```python
from build123d import *

# Parameters (mm, degrees)
SKETCH1_R           = 4.5
BOSS_EXTRUDE1_DEPTH = 4.5
SKETCH2_W           = 8
SKETCH2_H           = 10
BOSS_EXTRUDE2_DEPTH = 4.5
BOSS_EXTRUDE3_START = 4.5
SKETCH3_R           = 4.5
BOSS_EXTRUDE3_DEPTH = 4.5
FILLET3_R           = 5
FILLET4_R           = 5
SKETCH6_R           = 4.25
SKETCH6_R_2         = 1.5
BOSS_EXTRUDE4_DEPTH = 4.5
BOSS_EXTRUDE5_START = 4.5
SKETCH7_R           = 4.25
SKETCH7_R_2         = 1.5
BOSS_EXTRUDE5_DEPTH = 4.5
BOSS_EXTRUDE6_START = -2
SKETCH8_R           = 4.25
BOSS_EXTRUDE6_DEPTH = 2
BOSS_EXTRUDE7_START = -9.5
SKETCH9_R           = 4.5
BOSS_EXTRUDE7_DEPTH = 9.5


with BuildPart() as part:
    # Sketch1 → Boss-Extrude1 (new body)
    with BuildSketch(Plane.XY):
        with BuildLine():
            Line((-15, 17.5), (-15, -14.5))
            Line((-15, -14.5), (-12, -14.5))
            Line((-12, -14.5), (-12, -17.5))
            Line((-12, -17.5), (12, -17.5))
            Line((12, -17.5), (12, -14.5))
            Line((12, -14.5), (15, -14.5))
            Line((15, -14.5), (15, 17.5))
            ThreePointArc((15, 17.5), (0, 26.843803595), (-15, 17.5))
        make_face()
        with Locations((0, 17.5)):
            Circle(SKETCH1_R, mode=Mode.SUBTRACT)
    extrude(amount=-BOSS_EXTRUDE1_DEPTH)

    # Sketch2 → Boss-Extrude2 (add)
    with BuildSketch(Plane(origin=(0, -17.5, 0), x_dir=(1, 0, 0), z_dir=(0, 1, 0))):
        Polygon((-12, 4.5), (12, 4.5), (12, 0), (12, -3), (15, -3), (15, -12.000675804), (22.5, -12.000675804), (22.5, -15.000675804), (25.5, -15.000675804), (30, -15.000675804), (30, -39.000675804), (25.5, -39.000675804), (22.5, -39.000675804), (22.5, -42.000675804), (15, -42.000675804), (15, -47.001351609), (12, -47.001351609), (12, -50), (12, -54.5), (-12, -54.5), (-12, -50), (-12, -47), (-15, -47), (-15, -42.000675804), (-22.5, -42.000675804), (-22.5, -39.000675804), (-25.5, -39.000675804), (-30, -39.000675804), (-30, -15.000675804), (-25.5, -15.000675804), (-22.5, -15.000675804), (-22.5, -12.000675804), (-15, -12.000675804), (-15, -3), (-12, -3), (-12, 0), align=None)
        with Locations((0, -27.000675804)):
            Rectangle(SKETCH2_W, SKETCH2_H, mode=Mode.SUBTRACT)
    extrude(amount=-BOSS_EXTRUDE2_DEPTH)

    # Sketch3 → Boss-Extrude3 (add)
    with BuildSketch(Plane.XY.offset(50).offset(BOSS_EXTRUDE3_START)):
        with BuildLine():
            Line((-15, 17.5), (-15, -14.5))
            Line((-15, -14.5), (-12, -14.5))
            Line((-12, -14.5), (-12, -17.5))
            Line((-12, -17.5), (12, -17.5))
            Line((12, -17.5), (12, -14.5))
            Line((12, -14.5), (15, -14.5))
            Line((15, -14.5), (15, 17.5))
            ThreePointArc((15, 17.5), (0, 26.843803595), (-15, 17.5))
        make_face()
        with Locations((0, 17.5)):
            Circle(SKETCH3_R, mode=Mode.SUBTRACT)
    extrude(amount=-BOSS_EXTRUDE3_DEPTH)

    # Fillet3
    fillet3_edges = [part.edges().sort_by_distance(p)[0] for p in [
        (0, -22, 54.5),
    ]]
    fillet(fillet3_edges, radius=FILLET3_R)

    # Fillet4
    fillet4_edges = [part.edges().sort_by_distance(p)[0] for p in [
        (0, -22, -4.5),
    ]]
    fillet(fillet4_edges, radius=FILLET4_R)

    # Sketch6 → Boss-Extrude4 (add)
    with BuildSketch(Plane(origin=(-25.5, 0, 0), x_dir=(0, 0, -1), z_dir=(1, 0, 0))):
        Polygon((-15.000675804, -22), (-39.000675804, -22), (-39.000675804, -25), (-42.000675804, -25), (-42.000675804, -67), (-27.000675804, -75), (-12.000675804, -67), (-12.000675804, -25), (-15.000675804, -25), align=None)
        with Locations((-27.000675804, -49)):
            Circle(SKETCH6_R, mode=Mode.SUBTRACT)
        with Locations((-27.000675804, -61)):
            Circle(SKETCH6_R_2, mode=Mode.SUBTRACT)
    extrude(amount=-BOSS_EXTRUDE4_DEPTH)

    # Sketch7 → Boss-Extrude5 (add)
    with BuildSketch(Plane(origin=(25.5, 0, 0), x_dir=(0, 0, -1), z_dir=(1, 0, 0)).offset(BOSS_EXTRUDE5_START)):
        Polygon((-39.000675804, -22), (-39.000675804, -25), (-42.000675804, -25), (-42.000675804, -67), (-27.000675804, -75), (-12.000675804, -67), (-12.000675804, -25), (-15.000675804, -25), (-15.000675804, -22), align=None)
        with Locations((-27.000675804, -49)):
            Circle(SKETCH7_R, mode=Mode.SUBTRACT)
        with Locations((-27.000675804, -61)):
            Circle(SKETCH7_R_2, mode=Mode.SUBTRACT)
    extrude(amount=-BOSS_EXTRUDE5_DEPTH)

    # Sketch8 → Boss-Extrude6 (add)
    with BuildSketch(Plane.ZY.offset(30).offset(BOSS_EXTRUDE6_START)):
        with Locations(Location((27.000675804, -49, 0), (0, 0, 180))):
            Circle(SKETCH8_R)
    extrude(amount=BOSS_EXTRUDE6_DEPTH)

    # Sketch9 → Boss-Extrude7 (add)
    with BuildSketch(Plane(origin=(0, 0, 50), x_dir=(-1, 0, 0), z_dir=(0, 0, -1)).offset(BOSS_EXTRUDE7_START)):
        with Locations(Location((0, 17.5, 0), (0, 0, 180))):
            Circle(SKETCH9_R)
    extrude(amount=BOSS_EXTRUDE7_DEPTH)


solid = part.part
```
Read the model definition and answer for the solid it produces. Units are mm, in the model's axes. A direction names the side the tool comes from. Give positions to 0.01 mm unless a question says otherwise; leave off trailing zeros. Write each loop counter-clockwise with the first axis right and the second up, starting at its lowest first coordinate (ties: lowest second). Pieces come first, ordered by that corner, then holes. Notation, with made-up numbers: (32.25, 31) -> (63.25, 31) arc R13 ccw to (63.25, 43) -> close; hole circle Ø10 at (-11, -38.75). An arc over 180 degrees is marked (long way). Answer as a JSON object with one key per item and string values.
1) Section C-C on y = -23.5 is taken. Write down the section's boundary in (x, z).
Findings below:
{"outline": "(-30, 15) -> (-25.5, 15) -> (-25.5, 39) -> (-30, 39) -> close; (25.5, 15) -> (30, 15) -> (30, 39) -> (25.5, 39) -> close"}
2) Flat-ended cylindrical pins translate along their axes: pin 1 Ø4 at (y, z) = (-48.5, 28.5) entering from +X; pin 2 Ø3.5 at (x, y) = (-0.5, -19.5) entering from +Z; pin 3 Ø8 at (x, z) = (-10.5, 53) entering from +Y; pin 4 Ø4 at (x, y) = (23, -46.5) entering from +Z. Find the tip coordinate at first contact, or state that the pin passes through.
Findings below:
{"pin 1": "stops at x = -28", "pin 2": "stops at z = 54.44", "pin 3": "stops at y = 25.53", "pin 4": "passes through"}
3) Section D-D on z = 36 is taken. Write down the section's boundary in (x, y).
Findings below:
{"outline": "(-30, -70.2) -> (-25.5, -70.2) -> (-25.5, -22) -> (25.5, -22) -> (25.5, -70.2) -> (30, -70.2) -> (30, -17.5) -> (-30, -17.5) -> close"}
4) Section A-A on x = 0 is taken. Write down the section's boundary in (y, z), then the cut area to 3 significant figures.
Findings below:
{"outline": "(-22, 0.5) arc R5 ccw to (-17, -4.5) -> (13, -4.5) -> (13, 0) -> (-17.5, 0) -> (-17.5, 22) -> (-22, 22) -> close; (-22, 32) -> (-17.5, 32) -> (-17.5, 50) -> (26.84, 50) -> (26.84, 54.5) -> (22, 54.5) -> (22, 59.5) -> (13, 59.5) -> (13, 54.5) -> (-17, 54.5) arc R5 ccw to (-22, 49.5) -> close; (22, -4.5) -> (26.84, -4.5) -> (26.84, 0) -> (22, 0) -> close", "area": "613 mm^2"}
5) A tool of negligible diameter and unlimited length cuts with its end or side. For faces 4 (the flat face through (22.5, -20, 13)), 5 (the flat face through (-12, -18, -1)), 6 (the cylindrical face through (-26.73, -51.59, 30.37)), 7 (the flat face through (28, -25, 13)), 8 (the flat face through (-12, -18, 51)), from which of +Z, -Z, +X, -X, +Y, -Y can it reach the whole face along a straight path? Write none if from no direction.
Findings below:
{"face 4": "-Z, +X, +Y, -Y", "face 5": "-Z, -X, -Y", "face 6": "+X", "face 7": "-Z, +X, -X, +Y", "face 8": "+Z, -X, -Y"}
6) Straight lines are drawn through the part: probe 1 along X at (y, z) = (-48, 40); probe 2 along Z at (x, y) = (-4, -13); probe 3 along Z at (x, y) = (-27.35, -49). For each, find the intervals that lie inside material, in ascending order. Write a range as from..to.
Findings below:
{"probe 1": "x = -30..-25.5, 25.5..30", "probe 2": "z = -4.5..0, 50..54.5", "probe 3": "z = 12..22.75, 31.25..42"}
7) Section B-B on y = -57 is taken. Write down the section's boundary in (x, z).
Findings below:
{"outline": "(-30, 12) -> (-25.5, 12) -> (-25.5, 42) -> (-30, 42) -> close; (25.5, 12) -> (30, 12) -> (30, 42) -> (25.5, 42) -> close"}
8) For a pull along Z with two mould halves and no side action, classify faces 1 (the flat face through (28, -46, 42.001)), 2 (the cylindrical face through (-0.59, 13.04, 57.04)), 3 (the flat face through (0, 5, 0)) as pulls with the +Z half, pulls with the -Z half, needs draft (parallel to the pull), parting line crosses it, or undercut.
Findings below:
{"face 1": "pulls with the +Z half", "face 2": "needs draft", "face 3": "undercut"}
